Autodesk Fusion 360 part; units mm, degrees
sketch "Sketch1" plane through (0, 0, 0) normal (0, 0, 1) x (1, 0, 0)
  line L0 (3, 0) -> (61, 0)
  line L1 (64, 3) -> (64, 90)
  line L2 (61, 93) -> (3, 93)
  line L3 (0, 90) -> (0, 3)
  arc A0 (3, 93) -> (0, 90) centre (3, 90) ccw
  arc A1 (64, 90) -> (61, 93) centre (61, 90) ccw
  arc A2 (61, 0) -> (64, 3) centre (61, 3) ccw
  arc A3 (0, 3) -> (3, 0) centre (3, 3) ccw
  point P0 (64, 0)
  point P1 (0, 93)
  dimension "d1" = 64
  dimension "d2" = 93
  dimension "d3" = 3
  dimension "d4" = 3
extrude "Extrude1" add sketch "Sketch1" along normal blind 3
sketch "Sketch4" plane through (0, 0, 3) normal (0, 0, 1) x (-1, 0, 0)
  arc A0 (0, -3) -> (-3, 0) centre (-3, -3) ccw
  line L0 (-3, 0) -> (-61, 0)
  arc A1 (-61, 0) -> (-64, -3) centre (-61, -3) ccw
  line L1 (-64, -3) -> (-64, -90)
  arc A2 (-64, -90) -> (-61, -93) centre (-61, -90) ccw
  line L2 (-61, -93) -> (-3, -93)
  arc A3 (-3, -93) -> (0, -90) centre (-3, -90) ccw
  line L3 (0, -90) -> (0, -3)
  line L4 (-3, -3) -> (-61, -3)
  line L5 (-61, -3) -> (-61, -90)
  line L6 (-61, -90) -> (-3, -90)
  line L7 (-3, -90) -> (-3, -3)
  dimension "d11" = 58
  dimension "d12" = 87
  dimension "d13" = 3
  dimension "d14" = 3
extrude "Extrude2" add sketch "Sketch4" along normal blind 35
sketch "Sketch5" plane through (0, 0, 0) normal (0, -1, 0) x (1, 0, 0)
  line L0 (3, 0) -> (61, 0)
  line L1 (61, 0) -> (61, 23)
  line L2 (3, 23) -> (61, 23)
  line L3 (6, 6.8) -> (22.5, 6.8)
  line L4 (22.5, 6.8) -> (22.5, 23.8)
  line L5 (22.5, 23.8) -> (6, 23.8)
  line L6 (6, 23.8) -> (6, 6.8)
  line L7 (3, 0) -> (3, 23)
  line L8 (25.5, 23.8) -> (40.45, 23.8)
  line L9 (40.45, 23.8) -> (40.45, 6.8)
  line L10 (40.45, 6.8) -> (25.5, 6.8)
  line L11 (25.5, 6.8) -> (25.5, 23.8)
  line L12 (43.45, 6.8) -> (58.4, 6.8)
  line L13 (58.4, 6.8) -> (58.4, 23.8)
  line L14 (58.4, 23.8) -> (43.45, 23.8)
  line L15 (43.45, 23.8) -> (43.45, 6.8)
  line L16 (3, 0) -> (61, 0)
  line L17 (61, 0) -> (61, 38)
  line L18 (61, 38) -> (3, 38)
  line L19 (3, 38) -> (3, 0)
  dimension "d21" = 16.5
  dimension "d22" = 17
  dimension "d23" = 3
  dimension "d26" = 14.95
  dimension "d27" = 17
  dimension "d29" = 14.95
  dimension "d30" = 17
  dimension "d31" = 3
  dimension "d34" = 3
  dimension "d45" = 6.8
extrude "Extrude4" cut sketch "Sketch5" against normal blind 3 contours L2 L4 L5 L6 | L2 L3 L4 L6 | L2 L12 L13 L15 | L2 L13 L14 L15 | L2 L8 L9 L11 | L2 L9 L10 L11
sketch "Sketch6" plane through (0, 0, 3) normal (0, 0, 1) x (-1, 0, 0)
  line L0 (-3, -3) -> (-61, -3)
  line L1 (-61, -3) -> (-61, -90)
  line L2 (-61, -90) -> (-3, -90)
  line L3 (-3, -90) -> (-3, -3)
  circle A0 centre (-7.5, -85.5) radius 1
  circle A1 centre (-7.5, -85.5) radius 3
  circle A2 centre (-56.5, -85.5) radius 1
  circle A3 centre (-56.5, -85.5) radius 3
  circle A4 centre (-56.5, -27.5) radius 1
  circle A5 centre (-56.5, -27.5) radius 3
  circle A6 centre (-7.5, -27.5) radius 1
  circle A7 centre (-7.5, -27.5) radius 3
  dimension "d35" = 2
  dimension "d36" = 4.5
  dimension "d37" = 4.5
  dimension "d38" = 6
  dimension "d59" = 2
  dimension "d60" = 4.5
  dimension "d61" = 4.5
  dimension "d62" = 6
  dimension "d63" = 2
  dimension "d64" = 4.5
  dimension "d65" = 58
  dimension "d66" = 6
  dimension "d67" = 2
  dimension "d68" = 4.5
  dimension "d69" = 58
  dimension "d70" = 6
extrude "Extrude6" cut sketch "Sketch6" against normal blind 3 contours A0 | A2 | A4 | A6
extrude "Extrude7" add sketch "Sketch6" along normal blind 0.5 contours A1
sketch "Sketch7" plane through (0, 0, 0) normal (-1, 0, 0) x (0, -1, 0)
  line L0 (-90, 0) -> (-3, 0)
  line L1 (-3, 0) -> (-3, 38)
  line L2 (-3, 38) -> (-90, 38)
  line L3 (-90, 38) -> (-90, 0)
  line L4 (-88, 5) -> (-43, 5)
  line L5 (-43, 5) -> (-43, 16)
  line L6 (-43, 16) -> (-88, 16)
  line L7 (-88, 16) -> (-88, 5)
  dimension "d46" = 45
  dimension "d47" = 11
  dimension "d50" = 5
extrude "Extrude8" cut sketch "Sketch7" against normal blind 3 contours L4 L5 L6 L7
sketch "Sketch8" plane through (0, 93, 0) normal (0, 1, 0) x (-1, 0, 0)
  line L0 (-61, 0) -> (-3, 0)
  line L1 (-3, 0) -> (-3, 38)
  line L2 (-3, 38) -> (-61, 38)
  line L3 (-61, 38) -> (-61, 0)
  line L4 (-44.5, 3) -> (-19.5, 3)
  line L5 (-19.5, 3) -> (-19.5, 11)
  line L6 (-19.5, 11) -> (-44.5, 11)
  line L7 (-44.5, 11) -> (-44.5, 3)
  line L8 (-3, 0) -> (-3, 23)
  line L9 (-3, 0) -> (-61, 0)
  dimension "d51" = 25
  dimension "d52" = 8
  dimension "d53" = 16.5
  dimension "d54" = 3
extrude "Extrude9" cut sketch "Sketch8" against normal blind 3 contours L4 L5 L6 L7
extrude "Extrude10" add 1 faces at (9.6751, 86.3269, 3.5) along direction (0, 0, 1) blind 1.5
extrude "Extrude11" add sketch "Sketch6" along normal blind 2 contours A3 | A5 | A7
extrude "Extrude13" add sketch "Sketch6" along normal blind 3 contours A4
extrude "Extrude14" add sketch "Sketch6" along normal blind 3 contours A0 | A2 | A6
sketch "Sketch11" plane through (0, 0, 0) normal (-1, 0, 0) x (0, -1, 0)
  line L0 (-43, 5) -> (-88, 5)
  line L1 (-88, 5) -> (-88, 16)
  line L2 (-88, 16) -> (-43, 16)
  line L3 (-43, 16) -> (-43, 5)
  line L4 (-90, 0) -> (-3, 0)
  line L5 (-3, 0) -> (-3, 38)
  line L6 (-3, 38) -> (-90, 38)
  line L7 (-90, 38) -> (-90, 0)
  line L8 (-81.3, 38) -> (-59.3, 38)
  line L9 (-59.3, 38) -> (-59.3, 22)
  line L10 (-59.3, 22) -> (-81.3, 22)
  line L11 (-81.3, 22) -> (-81.3, 38)
  dimension "d85" = 22
  dimension "d86" = 16
  dimension "d87" = 8.7
extrude "Extrude15" cut sketch "Sketch11" against normal blind 3 contours L6 L8 L9 L10 L11
fillet "Fillet1" radius 1 1 edges at (1.5, 81.3, 22)
fillet "Fillet2" radius 1 21 edges at (1.5, 59.3, 22) (44.5, 91.5, 3) (44.5, 91.5, 11) (19.5, 91.5, 3) (19.5, 91.5, 11) (1.5, 43, 5) (6, 1.5, 6.8) (25.5, 1.5, 6.8) (43.45, 1.5, 6.8) (6, 1.5, 23.8) (25.5, 1.5, 23.8) (43.45, 1.5, 23.8) (40.45, 1.5, 23.8) (22.5, 1.5, 23.8) (58.4, 1.5, 23.8) (1.5, 88, 16) (1.5, 88, 5) (22.5, 1.5, 6.8) (40.45, 1.5, 6.8) (58.4, 1.5, 6.8) (1.5, 43, 16)
delete_face "DeleteFace1" 1 faces at (1, 80.5358, 22.0282)
delete_face "DeleteFace2" 1 faces at (1, 59.8, 22.134)
Geometry: final body of the model. Coordinates: model frame, mm. A direction names the side the tool comes from. Coordinates: 2 decimals unless noted, no trailing zeros. Loops run counter-clockwise (first coordinate to the right, second up) from the corner with the lowest first, then second, coordinate; pieces in that order, holes last. Notation, with made-up numbers: (41.25, 38.5) - (48.25, 38.5) arc R16 cw to (48.25, 48.5) - close; hole circle Ø11 at (24, 72). An arc over 180 degrees is marked (long way). Put each result on its own line as item: value. Start each with the question number.
Q1. Cut plane D-D, the plane z = 28.5. Return loops of the section in (x, y).
Q2. Line query: line 1 (Y direction, x = 7.5, z = 0.8); line 2 (X direction, y = 27.5, z = 1.1); line 3 (Y direction, x = 27, z = 24.5). Output: solid intervals per line, ascending.
Q3. Pull-direction query (Y, two-part tool) for faces 5 (the flat face through (8, 85, 6)), 6 (the flat face through (25.5, 1, 15)), 7 (the cylindrical face through (0.86, 92.1, 18.73)); classes: released by +Y, released by -Y, zero draft, split by the parting line, or undercut.
Q4. Pin query (flat end, axial travel): pin 1 Ø2 at (x, y) = (7, 85.5) entering from +Z; pin 2 Ø0.9 at (x, z) = (1, 33.5) entering from +Y; pin 3 Ø1.5 at (x, z) = (1.5, 33) entering from -Y. Return the tip coordinate at first contact, or that it passes through.
Q5. Cut plane A-A, the plane x = 16. Return loops of the section in (y, z), and give its area (3 significant figures).
Q6. Cut plane C-C, the plane y = 11. Return loops of the section in (x, z).
Q7. Cut plane B-B, the plane y = 66.5. Return loops of the section in (x, z).
Q8. Set-up query: faces 1 (the flat face through (57, 85, 6)), 2 (the flat face through (14, 1, 6.8)), 3 (the cylindrical face through (7.63, 26.51, 1.52)), 4 (the flat face through (8, 29, 5)). Return all of +Z, -Z, +X, -X, +Y, -Y with unobstructed straight access to the full face (end or side cutting, diameter ignored); none if empty.
Filled sheet:
1. outline: (0, 3) arc R3 ccw to (3, 0) - (61, 0) arc R3 ccw to (64, 3) - (64, 90) arc R3 ccw to (61, 93) - (3, 93) arc R3 ccw to (0, 90) - (0, 81.3) - (3, 81.3) - (3, 90) - (61, 90) - (61, 3) - (3, 3) - (3, 59.3) - (0, 59.3) - close
2. line 1: 0 to 26.5, 28.5 to 84.5, 86.5 to 93
2. line 2: 0 to 6.5, 8.5 to 55.5, 57.5 to 64
2. line 3: 0 to 3, 90 to 93
3. face 5: undercut
3. face 6: zero draft
3. face 7: released by +Y
4. pin 1: z = 6
4. pin 2: y = 92.57
4. pin 3: y = 0.1
5. outline: (0, 0) - (93, 0) - (93, 38) - (90, 38) - (90, 3) - (3, 3) - (3, 6.8) - (0, 6.8) - close; (0, 23.8) - (3, 23.8) - (3, 38) - (0, 38) - close
5. area: 438 mm²
6. outline: (0, 0) - (64, 0) - (64, 38) - (61, 38) - (61, 3) - (3, 3) - (3, 38) - (0, 38) - close
7. outline: (0, 0) - (64, 0) - (64, 38) - (61, 38) - (61, 3) - (3, 3) - (3, 5) - (0, 5) - close; (0, 16) - (3, 16) - (3, 22) - (0, 22) - close
8. face 1: +Z, -X
8. face 2: -Y
8. face 3: -Z
8. face 4: +Z
